```python
from build123d import *

# Parameters (mm, degrees)
CYLINDER005_R     = 6.5
CYLINDER005_DEPTH = 2
SKETCH003_R       = 2.1
EXTRUDE004_DEPTH  = 2


with BuildPart() as motormountcutout:
    # Cylinder005 → Cylinder005 (new body)
    with BuildSketch(Plane(origin=(0, 0, 8), x_dir=(1, 0, 0), z_dir=(0, -1, 0))):
        Circle(CYLINDER005_R)
    extrude(amount=CYLINDER005_DEPTH)


with BuildPart() as motormount:
    # Sketch003 → Extrude004 (new body)
    with BuildSketch(Plane.XZ):
        with BuildLine():
            ThreePointArc((-17.500023, 3.5), (-19.97489, 2.474858), (-21, -2.3e-05))
            Line((-21, -2.3e-05), (-21, -12.500023))
            Line((-21, -12.500023), (21, -12.500023))
            Line((21, 0), (21, -12.500023))
            ThreePointArc((21, 0), (19.974874, 2.474874), (17.5, 3.5))
            Line((-17.500023, 3.5), (17.5, 3.5))
        make_face()
        with Locations((17.5, 0)):
            Circle(SKETCH003_R, mode=Mode.SUBTRACT)
        with Locations((-17.5, 0)):
            Circle(SKETCH003_R, mode=Mode.SUBTRACT)
    extrude(amount=EXTRUDE004_DEPTH)

    # Cut004: cut motorMountCutout
    add(motormountcutout.part, mode=Mode.SUBTRACT)


with BuildPart() as motormount_1:
    # Cut004 placement: moved
    add(motormount.part.moved(Location((0, 0, -8))))


solid = motormount_1.part
```
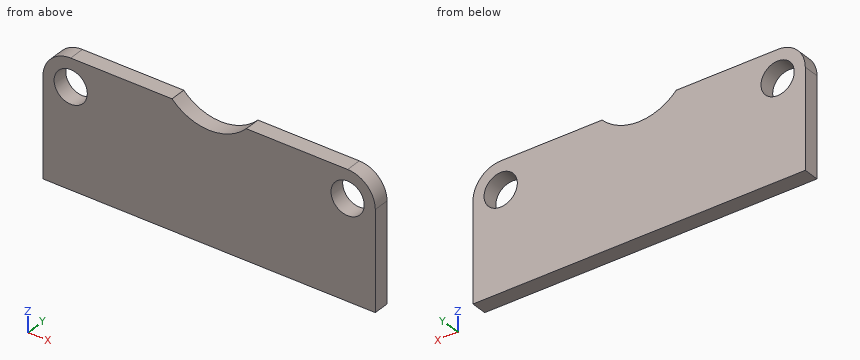
Model file for the job. Use its own axes, mm. Give positions to 0.01 mm unless a question says otherwise; leave off trailing zeros. Order: outer loops, then holes, each group sorted by start corner. A loop starts at its lowest first (then second) coordinate and runs counter-clockwise, first axis right, second up.
1) Saw through at D-D, the plane x = -2. Write the cut outline in (y, z).
2) Saw through at B-B, the plane x = 16. Write the cut outline in (y, z), then the cut area to 3 significant figures.
3) Saw through at C-C, the plane z = -9.5. Write the cut outline in (x, y), then the cut area to 3 significant figures.
4) Saw through at A-A, the plane y = -0.8. Write the cut outline in (x, z), then the cut area to 3 significant figures.
5) Wall check: probe 1 along Z at (x, y) = (-17.5, -1.15); probe 2 along X at (y, z) = (-1.4, -7.5); probe 3 along Z at (x, y) = (18, -1.15). Give the ranges that are in metal, low to high.
Computed:
1. outline: (-2, -20.5) - (0, -20.5) - (0, -6.18) - (-2, -6.18) - close
2. outline: (-2, -20.5) - (0, -20.5) - (0, -9.47) - (-2, -9.47) - close; (-2, -6.53) - (0, -6.53) - (0, -4.5) - (-2, -4.5) - close
2. area: 26.1 mm2
3. outline: (-21, -2) - (-18.97, -2) - (-18.97, 0) - (-21, 0) - close; (-16.03, -2) - (16.03, -2) - (16.03, 0) - (-16.03, 0) - close; (18.97, -2) - (21, -2) - (21, 0) - (18.97, 0) - close
3. area: 72.2 mm2
4. outline: (-21, -20.5) - (21, -20.5) - (21, -8) arc R3.5 ccw to (17.5, -4.5) - (4.69, -4.5) arc R6.5 cw to (-4.69, -4.5) - (-17.5, -4.5) arc R3.5 ccw to (-21, -8) - close; hole circle Ø4.2 at (-17.5, -8); hole circle Ø4.2 at (17.5, -8)
4. area: 626 mm2
5. probe 1: z = -20.5 to -10.1, -5.9 to -4.5
5. probe 2: x = -20.96 to -19.54, -15.46 to 15.46, 19.54 to 20.96
5. probe 3: z = -20.5 to -10.04, -5.96 to -4.54
